The listing builds one solid part. Answer for the finished solid, in the listing's coordinates (mm). A direction names the side the tool comes from. Coordinates: 2 decimals unless noted, no trailing zeros. Order: outer loops, then holes, each group sorted by start corner. A loop starts at its lowest first (then second) coordinate and runs counter-clockwise, first axis right, second up. Notation, with made-up numbers: (7, -6) -> (56, -6) arc R26 ccw to (56, 20) -> close; hole circle Ø3 at (45.25, 16). An arc over 180 degrees is marked (long way). Write each question's results on one line, items separated by ' | '. Start each with the question number.
(1) The part is cut by section C-C, the plane z = -7.5. Give the vertices of the cut face in (x, y).
(2) The part is cut by section D-D, the plane y = 3.75. Give the vertices of the cut face in (x, z).
(3) A tool of negligible diameter and unlimited length cuts with its end or side. For faces 1 (the face through (-5, 7, 0)), 2 (the face through (-1, 7, -5.6)), 3 (the face through (6, 7, -10.6)), 4 (the face through (10, 2, -10)), 5 (the face through (-3.5, 5, 6)), from which of +Z, -Z, +X, -X, +Y, -Y can it reach the whole face along a straight path? Write none if from no direction.
(4) The part is cut by section A-A, the plane z = 6.1. Give the vertices of the cut face in (x, y), then the cut area to 3 significant figures.
(5) Straight lines are drawn through the part: L1, parallel to X at y = 7.5, z = -1.5; L2, parallel to Z at x = 7, y = 12.75; L3, parallel to X at y = 3.75, z = 5.75. For each, find the intervals that lie inside material, in ascending order.
(6) Determine the mould class of faces 6 (the face through (6, 14, -3)), 7 (the face through (0, 7, -3.6)), 8 (the face through (5, 7, 8.6)) for opening direction Z: +Z half, -Z half, draft (parallel to the pull), parting line (faces both ways), or undercut.
(7) Given pin 1 (0.8 mm diameter, centred on x = -4, y = 9.5, fed in from -Z); pin 2 (1.6 mm diameter, centred on x = 10.5, y = 13, fed in from +Z); pin 3 (2 mm diameter, centred on y = 6, z = 2, fed in from +X); pin 4 (2.5 mm diameter, centred on y = 7, z = 6.1, fed in from -X), each flat-ended and moving along its own axis, determine where each tip first touches the part or whether it passes through.
(8) The part is cut by section B-B, the plane x = 9. Give the vertices of the cut face in (y, z), then the cut area to 3 significant figures.
Autodesk Inventor part; units mm, degrees
ref_plane "YZ Plane" through (0, 0, 0) normal (1, 0, 0) x (0, 1, 0)
ref_plane "XZ Plane" through (0, 0, 0) normal (0, 1, 0) x (-1, 0, 0)
ref_plane "XY Plane" through (0, 0, 0) normal (0, 0, 1) x (1, 0, 0)
sketch "Sketch1" plane through (0, 0, 0) normal (0, 1, 0) x (-1, 0, 0)
  line L0 (5, 3.6) -> (-5, 3.6)
  line L1 (-5, 3.6) -> (-5, -3.6)
  line L2 (-5, -3.6) -> (5, -3.6)
  line L3 (5, -3.6) -> (5, 3.6)
  line L4 (6.5, 8.6) -> (6.5, -5.6)
  line L5 (6.5, -5.6) -> (-6.5, -5.6)
  line L6 (-6.5, -5.6) -> (-6.5, 8.6)
  line L7 (-6.5, 8.6) -> (-3.5, 8.6)
  line L8 (6.5, 8.6) -> (3.5, 8.6)
  line L9 (3.5, 8.6) -> (3.5, 3.6)
  line L10 (-3.5, 8.6) -> (-3.5, 3.6)
  point P0 (0, 0)
  point P1 (5, 0)
  point P2 (0, -3.6)
  point P3 (-5, 8.6)
  point P4 (5, 8.6)
  dimension "d0" = 7.2
  dimension "d1" = 10
  dimension "d2" = 1.5
  dimension "d3" = 1.5
  dimension "d4" = 5
  dimension "d5" = 1.5
  dimension "d6" = 2
extrude "Extrusion1" add sketch "Sketch1" along normal blind 14 contours L0 L9 L8 L4 L5 L6 L7 L10 L1 L2 L3
sketch "Sketch2" plane through (6.5, 0, 8.6) normal (1, 0, 0) x (0, 0, -1)
  circle A0 centre (2.5, 7) radius 1.5
  line L0 (0, 0) -> (0, 14)
  point P0 (8.6, 0)
  point P1 (0, 7)
  dimension "d9" = 2.5
  dimension "d10" = 3
extrude "Extrusion2" cut sketch "Sketch2" against normal blind 14.75
sketch "Sketch3" plane through (6.5, 0, -5.6) normal (0, 0, -1) x (-1, 0, 0)
  line L0 (3, 0) -> (0, 0)
  line L1 (0, 0) -> (-6, 0)
  line L2 (-6, 0) -> (-6, 2)
  line L3 (-6, 2) -> (0, 2)
  line L4 (0, 2) -> (0, 0)
  line L5 (3, 14) -> (0, 14)
  line L6 (0, 14) -> (-6, 14)
  line L7 (-6, 14) -> (-6, 12)
  line L8 (-6, 12) -> (0, 12)
  line L9 (0, 12) -> (0, 14)
  line L10 (0, 0) -> (0, 14)
  point P0 (6.5, 0)
  point P1 (-6, 1)
  point P2 (-6, 13)
  dimension "d13" = 2
  dimension "d14" = 2
  dimension "d15" = 6
extrude "Extrusion3" add sketch "Sketch3" along normal mid plane 10
sketch "Sketch4" plane through (-6.5, 0, -5.6) normal (0, 0, -1) x (-1, 0, 0)
  line L0 (-13, 0) -> (-13, 14)
  line L1 (-10, 0) -> (-13, 0)
  line L2 (-13, 14) -> (-11, 14)
  line L3 (-11, 14) -> (-11, 0)
  line L4 (-11, 0) -> (-13, 0)
  line L5 (-13, 0) -> (-13, 14)
  point P0 (-6.5, 0)
  dimension "d18" = 2
extrude "Extrusion4" add sketch "Sketch4" along normal blind 5
sketch "Sketch5" plane through (0, 0, 0) normal (0, -1, 0) x (1, 0, 0)
  line L0 (12.5, -0.6) -> (12.5, -10.6)
  line L1 (6.5, -0.6) -> (6.5, -10.6)
  line L2 (12.5, -8.6) -> (6.5, -8.6)
  line L3 (6.5, -8.6) -> (6.5, -5.6)
  line L4 (6.5, -5.6) -> (12.5, -5.6)
  line L5 (12.5, -5.6) -> (12.5, -8.6)
  point P0 (0, 0)
  point P1 (9.5, -5.6)
  point P2 (4.5, -5.6)
  dimension "d21" = 3
extrude "Extrusion5" cut sketch "Sketch5" against normal blind 23.5
sketch "Sketch6" plane through (12.5, 0, -0.6) normal (1, 0, 0) x (0, 0, -1)
  line L0 (0, 0) -> (0, 2)
  line L1 (8, 14) -> (10, 14)
  line L2 (0, 0) -> (10, 0)
  line L3 (10, 0) -> (10, 14)
  line L4 (10, 14) -> (0, 14)
  line L5 (0, 14) -> (0, 0)
  point P0 (-0.6, 0)
extrude "Extrusion6" add sketch "Sketch6" along normal blind 2
properties part number "Frame_Clamp"
Established:
1) outline: (4.5, 0) -> (6.5, 0) -> (6.5, 14) -> (4.5, 14) -> close; (12.5, 0) -> (14.5, 0) -> (14.5, 14) -> (12.5, 14) -> close
2) outline: (-6.5, -5.6) -> (4.5, -5.6) -> (4.5, -10.6) -> (6.5, -10.6) -> (6.5, 8.6) -> (3.5, 8.6) -> (3.5, 3.6) -> (5, 3.6) -> (5, -3.6) -> (-5, -3.6) -> (-5, 3.6) -> (-3.5, 3.6) -> (-3.5, 8.6) -> (-6.5, 8.6) -> close; (12.5, -10.6) -> (14.5, -10.6) -> (14.5, -0.6) -> (12.5, -0.6) -> close
3) face 1: +Y, -Y | face 2: -Z, -X, +Y, -Y | face 3: -Z, +X, -X, +Y, -Y | face 4: +Z, -Z | face 5: +Z, +Y, -Y
4) outline: (-6.5, 0) -> (-3.5, 0) -> (-3.5, 5.5) -> (-6.5, 5.5) -> close; (-6.5, 8.5) -> (-3.5, 8.5) -> (-3.5, 14) -> (-6.5, 14) -> close; (3.5, 0) -> (6.5, 0) -> (6.5, 5.5) -> (3.5, 5.5) -> close; (3.5, 8.5) -> (6.5, 8.5) -> (6.5, 14) -> (3.5, 14) -> close | area: 66.0 mm^2
5) L1: x = -6.5 to -5, 5 to 6.5, 12.5 to 14.5 | L2: z = -10.6 to -8.6, -5.6 to -0.6 | L3: x = -6.5 to -3.5, 3.5 to 6.5
6) face 6: draft | face 7: undercut | face 8: +Z half
7) pin 1: stops at z = -5.6 | pin 2: stops at z = -0.6 | pin 3: stops at x = 6.5 | pin 4: passes through
8) outline: (0, -10.6) -> (2, -10.6) -> (2, -8.6) -> (0, -8.6) -> close; (0, -5.6) -> (2, -5.6) -> (2, -0.6) -> (0, -0.6) -> close; (12, -10.6) -> (14, -10.6) -> (14, -8.6) -> (12, -8.6) -> close; (12, -5.6) -> (14, -5.6) -> (14, -0.6) -> (12, -0.6) -> close | area: 28.0 mm^2
